Read the model definition and answer for the solid it produces. Units are mm, in the model's axes. Face numbers are marked on the shaded views. A direction names the side the tool comes from. Coordinates: 2 decimals unless noted, no trailing zeros. Loops run counter-clockwise (first coordinate to the right, second up) from the corner with the lowest first, then second, coordinate; pieces in that order, holes last. Notation, with made-up numbers: (75, 5.25) - (81, 5.25) arc R23 ccw to (81, 13.25) - close; hole circle Ø1 at (38.5, 28). An arc over 180 degrees is marked (long way). Use one line per item in the form item = value. Start each with the question number.
1) A cutting plane is placed at D-D (z = 2.95). Give the vertices of the cut face in (x, y), and give its area (3 significant figures).
2) A cutting plane is placed at B-B (x = 0). Give the vertices of the cut face in (y, z), and give its area (3 significant figures).
3) Each of these flat-tipped pins is pushed along its axis until it touches: P1, Ø1.6, axis at x = 0.5, y = -3.5, coming from the +Z side; P2, Ø1, axis at y = -4.5, z = 1.5, coming from the +X side; P3, Ø1.2, axis at x = 0.5, y = -4, coming from the +Z side; P4, Ø1.5, axis at x = 1.5, z = 0.5, coming from the +Y side. Where does it stop, or does it pass through?
4) Which of the six approach directions +Z, -Z, +X, -X, +Y, -Y give full straight-line access (tool end or side, diameter ignored) to the marked faces 1, 2, 3, 4 and 5?
5) Consider line 1 (Y direction, x = 3.75, z = 1.05); line 2 (Y direction, x = -1.5, z = 1.65). Determine where each line is inside the solid, lowest interval first.
6) A cutting plane is placed at C-C (y = -1). Give the vertices of the cut face in (x, z), and give its area (3 significant figures).
7) A cutting plane is placed at A-A (y = -5). Give the vertices of the cut face in (x, z), and give its area (3 significant figures).
from build123d import *

# Parameters (mm, degrees)
P_IDAT_VYSUNUT_M1_DEPTH  = 2.25
SKICA2_W                 = 3.5
SKICA2_H                 = 0.5
ODEBRAT_VYSUNUT_M1_DEPTH = 3.289126928
SKICA3_R                 = 4.4
P_IDAT_VYSUNUT_M2_DEPTH  = 1.89
SKICA5_W                 = 3.7
SKICA5_H                 = 1.288072418
ODEBRAT_VYSUNUT_M2_DEPTH = 2.89


with BuildPart() as part:
    # Skica1 → Přidat vysunutím1 (new body)
    with BuildSketch(Plane.XY):
        with BuildLine():
            Line((-2.3, -3.750999867), (-2.3, -5.730999867))
            Line((-2.3, -5.730999867), (2.3, -5.730999867))
            Line((2.3, -5.730999867), (2.3, -3.750999867))
            ThreePointArc((2.3, -3.750999867), (0, 4.4), (-2.3, -3.750999867))
        make_face()
    extrude(amount=P_IDAT_VYSUNUT_M1_DEPTH)

    # Skica2 → Odebrat vysunutím1 (cut)
    with BuildSketch(Plane(origin=(0, -5.730999867, 0), x_dir=(-1, 0, 0), z_dir=(0, -1, 0))):
        with Locations((0, -0.95)):
            Rectangle(SKICA2_W, SKICA2_H)
    extrude(amount=-ODEBRAT_VYSUNUT_M1_DEPTH, mode=Mode.SUBTRACT)

    # Skica3 → Přidat vysunutím2 (add)
    with BuildSketch(Plane.XY.offset(2.25)):
        with Locations(Location((0, 0, 0), (0, 0, 238.484629998))):
            Circle(SKICA3_R)
    extrude(amount=P_IDAT_VYSUNUT_M2_DEPTH)

    # Skica5 → Odebrat vysunutím2 (cut)
    with BuildSketch(Plane(origin=(0, -5.730999867, 0), x_dir=(-1, 0, 0), z_dir=(0, -1, 0))):
        with Locations((0, -4.395369221)):
            Rectangle(SKICA5_W, SKICA5_H)
    extrude(amount=-ODEBRAT_VYSUNUT_M2_DEPTH, mode=Mode.SUBTRACT)


solid = part.part
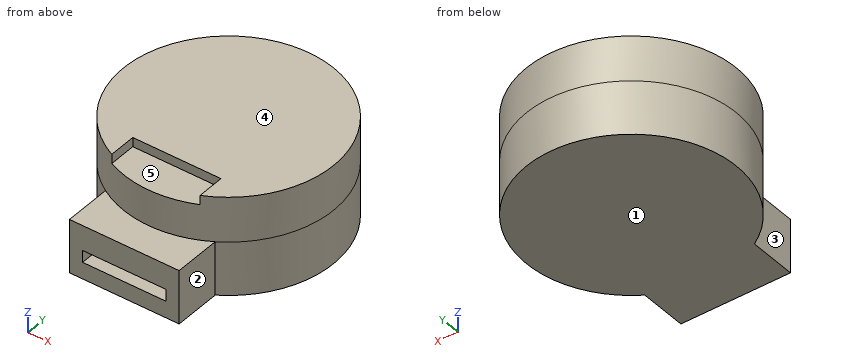
Found:
q1.outline = circle Ø8.8 at (0, 0)
q1.area = 60.8 mm^2
q2.outline = (-5.73, 0) - (4.4, 0) - (4.4, 4.14) - (-2.84, 4.14) - (-2.84, 3.75) - (-4.4, 3.75) - (-4.4, 2.25) - (-5.73, 2.25) - (-5.73, 1.2) - (-2.44, 1.2) - (-2.44, 0.7) - (-5.73, 0.7) - close
q2.area = 37.2 mm^2
q3.P1 = 4.14
q3.P2 = 2.3
q3.P3 = 3.75
q3.P4 = 4.34
q4.face_1 = -Z, +X, -X, +Y, -Y
q4.face_2 = +Z, -Z, +X, -Y
q4.face_3 = +Z, -Z, -X, -Y
q4.face_4 = +Z, +X, -X, +Y, -Y
q4.face_5 = +Z, -Y
q5.line_1 = -2.3 to 2.3
q5.line_2 = -5.73 to 4.14
q6.outline = (-4.28, 0) - (4.28, 0) - (4.28, 4.14) - (-4.28, 4.14) - close
q6.area = 35.5 mm^2
q7.outline = (-2.3, 0) - (2.3, 0) - (2.3, 2.25) - (-2.3, 2.25) - close; hole (-1.75, 0.7) - (1.75, 0.7) - (1.75, 1.2) - (-1.75, 1.2) - close
q7.area = 8.60 mm^2
